Source: CAD feature listing. Evaluate the final solid. Frame: model axes, mm. A direction names the side the tool comes from. Coordinates: 2 decimals unless noted, no trailing zeros. Loops run counter-clockwise (first coordinate to the right, second up) from the corner with the lowest first, then second, coordinate; pieces in that order, holes last. Notation, with made-up numbers: M 16,82 L 56,82 A27 cw 56,102 Z; hole C 60,5.25 d10. An arc over 180 degrees is marked long. One line per question, with ' | ' between items. Start each with the question number.
1. Mould query, pull axis X, two halves, no side actions, for faces 1 (the cylindrical face through (-31.03, 39.44, 13.9)), 2 (the flat face through (19.66, 39.44, 49.64)), 3 (the flat face through (-2, 39, 81.685)). Classes: pulls with the +X half, pulls with the -X half, needs draft (parallel to the pull), parting line crosses it, or undercut.
2. Ray query, probe 1 along X at (y, z) = (35.5, 56); probe 2 along X at (y, z) = (7, 28); probe 3 along Z at (x, y) = (4, 6.5) (3 decimals). Return the intervals inside material, ascending.
3. Access query for faces 4 (the flat face through (0, 5, 63)), 5 (the cylindrical face through (31.368, 39.44, 13.117)), 6 (the cylindrical face through (3.71, 39.44, 36.3)), 7 (the flat face through (32.247, 39.44, -17.174)). Directions: +Z, -Z, +X, -X, +Y, -Y. A direction counts if a zero-diameter tool reaches every point of the face in a straight line with its end or side. Return the directions, or none.
4. Section query C-C, the plane z = 20.5. Output: boundary loops of the cut face in (x, y).
5. Section query D-D, the plane z = 57. Output: boundary loops of the cut face in (x, y).
6. Section query A-A, the plane y = 10.5. Output: boundary loops of the cut face in (x, z) (3 decimals).
7. Pin query (flat end, axial travel): P1, Ø2.5, axis at x = 0, z = 66.5, coming from the +Y side; P2, Ø8, axis at x = -4.5, z = 31.5, coming from the +Y side; P3, Ø1, axis at x = 16.5, y = 29, coming from the +Z side; P4, Ø3, axis at y = 11, z = 29.5, coming from the +X side. Return the tip coordinate at first contact, or that it passes through.
8. Section query B-B, the plane x = 32.5. Output: boundary loops of the cut face in (y, z).
```python
from build123d import *

# Parameters (mm, degrees)
FIN_SLOT_EXTRUDE_DEPTH = 80
FIN_START              = -75
FIN_SLOT_DEPTH         = 75
FILLET1_R              = 10


with BuildPart() as part:
    # Sketch2 → Fin slot extrude (new body)
    with BuildSketch(Plane(origin=(0, 0, 0), x_dir=(1, 0, 0), z_dir=(0, 1, 0))):
        with BuildLine():
            Line((-35.253910446, -16.678183302), (-4.5, -81.685))
            Line((-4.5, -81.685), (4.5, -81.685))
            Line((4.5, -81.685), (35.253910446, -16.678183302))
            ThreePointArc((35.253910446, -16.678183302), (38.987980591, 0.968178408), (34.382638025, 18.407449646))
            Line((34.382638025, 18.407449646), (30.049957519, 15.90597539))
            ThreePointArc((30.049957519, 15.90597539), (0, -34), (-30.049957519, 15.90597539))
            Line((-30.049957519, 15.90597539), (-34.382638025, 18.407449646))
            ThreePointArc((-34.382638025, 18.407449646), (-38.987980591, 0.968178408), (-35.253910446, -16.678183302))
        make_face()
    extrude(amount=FIN_SLOT_EXTRUDE_DEPTH)

    # Sketch3 → Fin slot (cut)
    with BuildSketch(Plane(origin=(0, 80, 0), x_dir=(1, 0, 0), z_dir=(0, 1, 0)).offset(FIN_START)):
        with BuildLine():
            Line((1.6, -81.685), (1.6, -33.962332075))
            ThreePointArc((1.6, -33.962332075), (0, -34), (-1.6, -33.962332075))
            Line((-1.6, -33.962332075), (-1.6, -81.685))
            Line((-1.6, -81.685), (1.6, -81.685))
        make_face()
    extrude(amount=FIN_SLOT_DEPTH, mode=Mode.SUBTRACT)

    # Fillet1
    # the kernel refuses this fillet: 10 mm, written as the material it takes off along each edge
    with BuildSketch(Plane(origin=(-1.6, 5, 33.962332075), x_dir=(0, 0, 1), z_dir=(0, 1, 0))) as fillet1_piece_1:
        with BuildLine():
            CenterArc((8.481041966, -10), FILLET1_R, 90, 74.714058958)
            Line((-1.165179407, -7.363636364), (-1.358103835, -7.310909091))
            ThreePointArc((-1.358103835, -7.310909091), (-0.577691759, -3.682593204), (-0.199778424, 0.009411765))
            Line((-0.199778424, 0.009411765), (0, 0.2))
            Line((0, 0.2), (8.481041966, 0.2))
            Line((8.481041966, 0.2), (8.481041966, 0))
        make_face()
    extrude(amount=75, mode=Mode.SUBTRACT)
    with BuildSketch(Plane(origin=(1.6, 5, 33.962332075), x_dir=(0, 0, 1), z_dir=(0, 1, 0))) as fillet1_piece_2:
        with BuildLine():
            CenterArc((8.481041966, 10), FILLET1_R, 195.285941042, 74.714058958)
            Line((-1.165179407, 7.363636364), (-1.358103835, 7.310909091))
            ThreePointArc((-1.358103835, 7.310909091), (-0.577691759, 3.682593204), (-0.199778424, -0.009411765))
            Line((-0.199778424, -0.009411765), (0, -0.2))
            Line((0, -0.2), (8.481041966, -0.2))
            Line((8.481041966, -0.2), (8.481041966, 0))
        make_face()
    extrude(amount=75, mode=Mode.SUBTRACT)
    with BuildSketch(Plane(origin=(0, 5, 0), x_dir=(0.7049632922211216, 0, 0.7092437920918008), z_dir=(0.7092437920918008, 0, -0.7049632922211216))) as fillet1_piece_3_section:
        with BuildLine():
            CenterArc((34 + FILLET1_R, FILLET1_R), FILLET1_R, 180, 90)
            Line((34, FILLET1_R), (34 - FILLET1_R * 0.02, FILLET1_R))
            Line((34 - FILLET1_R * 0.02, FILLET1_R), (34 - FILLET1_R * 0.02, -FILLET1_R * 0.02))
            Line((34 - FILLET1_R * 0.02, -FILLET1_R * 0.02), (34 + FILLET1_R, -FILLET1_R * 0.02))
            Line((34 + FILLET1_R, -FILLET1_R * 0.02), (34 + FILLET1_R, 0))
        make_face()
    fillet1_piece_3 = revolve(axis=Axis((0, 5, 0), (0, -1, 0)), revolution_arc=89.653157122, mode=Mode.PRIVATE)
    fillet1_piece_3 = split(fillet1_piece_3, bisect_by=Plane(origin=(1.6, 2.736001805, 36.252063161), z_dir=(-1, 0, 0)), keep=Keep.TOP, mode=Mode.PRIVATE)
    fillet1_piece_3 = split(fillet1_piece_3, bisect_by=Plane(origin=(-1.6, 2.736001805, 36.252063161), z_dir=(1, 0, 0)), keep=Keep.TOP, mode=Mode.PRIVATE)
    add(fillet1_piece_3, mode=Mode.SUBTRACT)
    with BuildSketch(Plane(origin=(0, 5, 0), x_dir=(0.7049632922211216, 0, 0.7092437920918008), z_dir=(0.7092437920918008, 0, -0.7049632922211216))) as fillet1_piece_4a_section:
        with BuildLine():
            CenterArc((34 + FILLET1_R, FILLET1_R), FILLET1_R, 180, 90)
            Line((34, FILLET1_R), (34 - FILLET1_R * 0.02, FILLET1_R))
            Line((34 - FILLET1_R * 0.02, FILLET1_R), (34 - FILLET1_R * 0.02, -FILLET1_R * 0.02))
            Line((34 - FILLET1_R * 0.02, -FILLET1_R * 0.02), (34 + FILLET1_R, -FILLET1_R * 0.02))
            Line((34 + FILLET1_R, -FILLET1_R * 0.02), (34 + FILLET1_R, 0))
        make_face()
    fillet1_piece_4a = revolve(axis=Axis((0, 5, 0), (0, -1, 0)), revolution_arc=89.653157122, mode=Mode.PRIVATE)
    fillet1_piece_4a = split(fillet1_piece_4a, bisect_by=Plane(origin=(-1.6, 2.81629174, 32.584573329), z_dir=(-1, 0, 0)), keep=Keep.TOP, mode=Mode.PRIVATE)
    with BuildSketch(Plane(origin=(-1.6, -16.202604914, 33.962332075), x_dir=(0, 0, 1), z_dir=(0, 1, 0))) as fillet1_piece_4b_section:
        with BuildLine():
            CenterArc((8.481041966, -10), FILLET1_R, 90, 74.714058958)
            Line((-1.165179407, -7.363636364), (-1.358103835, -7.310909091))
            ThreePointArc((-1.358103835, -7.310909091), (-0.577691759, -3.682593204), (-0.199778424, 0.009411765))
            Line((-0.199778424, 0.009411765), (0, 0.2))
            Line((0, 0.2), (8.481041966, 0.2))
            Line((8.481041966, 0.2), (8.481041966, 0))
        make_face()
    fillet1_piece_4b = extrude(amount=96.202604914, mode=Mode.PRIVATE)
    fillet1_piece_4b = split(fillet1_piece_4b, bisect_by=Plane(origin=(-3.235617235, 5, 35.755925785), z_dir=(0, -1, 0)), keep=Keep.TOP, mode=Mode.PRIVATE)
    fillet1_piece_4 = fillet1_piece_4a & fillet1_piece_4b
    add(fillet1_piece_4, mode=Mode.SUBTRACT)
    with BuildSketch(Plane(origin=(1.6, -16.202604914, 33.962332075), x_dir=(0, 0, 1), z_dir=(0, 1, 0))) as fillet1_piece_5a_section:
        with BuildLine():
            CenterArc((8.481041966, 10), FILLET1_R, 195.285941042, 74.714058958)
            Line((-1.165179407, 7.363636364), (-1.358103835, 7.310909091))
            ThreePointArc((-1.358103835, 7.310909091), (-0.577691759, 3.682593204), (-0.199778424, -0.009411765))
            Line((-0.199778424, -0.009411765), (0, -0.2))
            Line((0, -0.2), (8.481041966, -0.2))
            Line((8.481041966, -0.2), (8.481041966, 0))
        make_face()
    fillet1_piece_5a = extrude(amount=96.202604914, mode=Mode.PRIVATE)
    fillet1_piece_5a = split(fillet1_piece_5a, bisect_by=Plane(origin=(3.235617235, 5, 35.755925785), z_dir=(0, -1, 0)), keep=Keep.TOP, mode=Mode.PRIVATE)
    with BuildSketch(Plane(origin=(0, 5, 0), x_dir=(0.7049632922211216, 0, 0.7092437920918008), z_dir=(0.7092437920918008, 0, -0.7049632922211216))) as fillet1_piece_5b_section:
        with BuildLine():
            CenterArc((34 + FILLET1_R, FILLET1_R), FILLET1_R, 180, 90)
            Line((34, FILLET1_R), (34 - FILLET1_R * 0.02, FILLET1_R))
            Line((34 - FILLET1_R * 0.02, FILLET1_R), (34 - FILLET1_R * 0.02, -FILLET1_R * 0.02))
            Line((34 - FILLET1_R * 0.02, -FILLET1_R * 0.02), (34 + FILLET1_R, -FILLET1_R * 0.02))
            Line((34 + FILLET1_R, -FILLET1_R * 0.02), (34 + FILLET1_R, 0))
        make_face()
    fillet1_piece_5b = revolve(axis=Axis((0, 5, 0), (0, -1, 0)), revolution_arc=89.653157122, mode=Mode.PRIVATE)
    fillet1_piece_5b = split(fillet1_piece_5b, bisect_by=Plane(origin=(1.6, 2.816291902, 32.584573464), z_dir=(1, 0, 0)), keep=Keep.TOP, mode=Mode.PRIVATE)
    fillet1_piece_5 = fillet1_piece_5a & fillet1_piece_5b
    add(fillet1_piece_5, mode=Mode.SUBTRACT)


solid = part.part
```
Taken from the geometry:
1) face 1: undercut | face 2: pulls with the +X half | face 3: needs draft
2) probe 1: -16.65 to -1.6, 1.6 to 16.65 | probe 2: -29.9 to -19.29, 19.29 to 29.9 | probe 3: 35.944 to 81.685
3) face 4: +Z, -Z, +Y | face 5: +Y, -Y | face 6: -Z, +Y | face 7: -Z, +Y, -Y
4) outline: M -33.45,0 L -27.12,0 L -27.12,80 L -33.45,80 Z; M 27.12,0 L 33.45,0 L 33.45,80 L 27.12,80 Z
5) outline: M -16.18,0 L 16.18,0 L 16.18,80 L 1.6,80 L 1.6,5 L -1.6,5 L -1.6,80 L -16.18,80 Z
6) outline: M -35.254,16.678 A39 ccw -34.383,-18.407 L -30.05,-15.906 A34 cw -8.964,32.797 A10 ccw -1.6,42.443 L -1.6,81.685 L -4.5,81.685 Z; M 1.6,42.443 A10 ccw 8.964,32.797 A34 cw 30.05,-15.906 L 34.383,-18.407 A39 ccw 35.254,16.678 L 4.5,81.685 L 1.6,81.685 Z
7) P1: y = 5 | P2: y = 80 | P3: z = 57.38 | P4: x = 29.9
8) outline: M 0,-17.32 L 80,-17.32 L 80,-9.99 L 0,-9.99 Z; M 0,9.99 L 80,9.99 L 80,22.5 L 0,22.5 Z
